Autodesk Inventor part; units mm, degrees
ref_plane "YZ Plane" through (0, 0, 0) normal (1, 0, 0) x (0, 1, 0)
ref_plane "XZ Plane" through (0, 0, 0) normal (0, 1, 0) x (-1, 0, 0)
ref_plane "XY Plane" through (0, 0, 0) normal (0, 0, 1) x (1, 0, 0)
sketch "Sketch1" plane through (0, 0, 0) normal (0, 1, 0) x (-1, 0, 0)
  line L0 (70, 50) -> (-70, 50)
  line L1 (-70, 50) -> (-70, -50)
  line L2 (-70, -50) -> (70, -50)
  line L3 (70, -50) -> (70, 50)
  line L4 (70, 50) -> (-70, -50) construction
  line L5 (-70, 50) -> (70, -50) construction
  point P0 (0, 0)
  dimension "d0" = 140
  dimension "d1" = 100
extrude "Extrusion1" add sketch "Sketch1" along normal blind 3.125
sketch "Sketch9" plane through (0, 3.125, 0) normal (0, 1, 0) x (1, 0, 0)
  circle A0 centre (-1.7146, 21.2758) radius 10
  point P0 (0, 0)
  dimension "d41" = 20
extrude "Extrusion9" cut sketch "Sketch9" against normal blind 10
sketch "Sketch10" plane through (0, 3.125, 0) normal (0, 1, 0) x (1, 0, 0)
  circle A0 centre (-31.6428, 0) radius 2
  point P0 (0, 0)
  dimension "d44" = 4
extrude "Extrusion10" cut sketch "Sketch10" against normal blind 5
sketch "Sketch11" plane through (0, 3.125, 0) normal (0, 1, 0) x (1, 0, 0)
  circle A0 centre (20.6742, 0) radius 2
  point P0 (0, 0)
  dimension "d47" = 4
extrude "Extrusion11" cut sketch "Sketch11" against normal blind 5
sketch "Sketch15" plane through (0, 3.125, 0) normal (0, 1, 0) x (1, 0, 0)
  line L0 (-16.402, 10) -> (-13.247, 10)
  line L1 (-13.247, 10) -> (-13.247, -10)
  line L2 (-13.247, -10) -> (-16.402, -10)
  line L3 (-16.402, -10) -> (-16.402, 10)
  line L4 (-16.402, 10) -> (-13.247, -10) construction
  line L5 (-13.247, 10) -> (-16.402, -10) construction
  line L6 (61.753, 10) -> (64.908, 10)
  line L7 (64.908, 10) -> (64.908, -10)
  line L8 (64.908, -10) -> (61.753, -10)
  line L9 (61.753, -10) -> (61.753, 10)
  line L10 (61.753, 10) -> (64.908, -10) construction
  line L11 (64.908, 10) -> (61.753, -10) construction
  point P0 (0, 0)
  point P1 (-14.8245, 0)
  point P2 (63.3305, 0)
  dimension "d68" = 3.155
  dimension "d69" = 20
  dimension "d70" = 3.155
  dimension "d71" = 20
  dimension "d72" = 75
extrude "Extrusion14" cut sketch "Sketch15" against normal blind 3.125
sketch "Sketch16" plane through (0, 3.125, 0) normal (0, 1, 0) x (1, 0, 0)
  line L0 (-70, -50) -> (70, -50)
  line L1 (-70, 50) -> (-40.7108, 50)
  line L2 (-40.7108, 50) -> (-40.7108, -50)
  line L3 (-40.7108, -50) -> (-70, -50)
  line L4 (-70, -50) -> (-70, 50)
  point P0 (0, 0)
extrude "Extrusion15" cut sketch "Sketch16" against normal blind 3.125
properties part number "Base"
The listing builds one solid part. Answer for the finished solid, in the listing's coordinates (mm). A direction names the side the tool comes from. Give positions to 0.01 mm unless a question says otherwise; leave off trailing zeros. Order: outer loops, then holes, each group sorted by start corner. A loop starts at its lowest first (then second) coordinate and runs counter-clockwise, first axis right, second up. Notation, with made-up numbers: (68, 83) - (97, 83) arc R34 ccw to (97, 119) - close; hole circle Ø6 at (74.25, 86). An arc over 180 degrees is marked (long way). Use one line per item in the form item = value. Start each with the question number.
(1) Consider line 1 (X direction, y = 0.75, z = 0); line 2 (X direction, y = 2.4, z = -7.5); line 3 (Z direction, x = 1, y = 0.35). Determine where each line is inside the solid, lowest interval first. Write a range as from..to.
(2) For faces 1 (the flat face through (70, 2, 1)), 2 (the flat face through (-15, 2, 10)), determine the directions among +Z, -Z, +X, -X, +Y, -Y from which every point of the face is accessible in a straight line to the end or side of a thin tool.
(3) A cutting plane is placed at B-B, the plane y = 2.6. Write down the section's boundary in (x, z), then the cut area to 3 significant figures.
(4) The mould has two halves that part along Z. Classify faces 3 (the flat face through (63, 2, -10)), 4 (the flat face through (-40.711, 2, -1)), 5 (the flat face through (61.753, 2, 0)), 6 (the flat face through (14, 2, 50)): released by +Z, released by -Z, zero draft, split by the parting line, or undercut.
(5) A cutting plane is placed at A-A, the plane z = 6. Write down the section's boundary in (x, y) (3 decimals), then the cut area to 3 significant figures.
Ans:
q1.line_1 = -40.71..-33.64, -29.64..-16.4, -13.25..18.67, 22.67..61.75, 64.91..70
q1.line_2 = -40.71..-16.4, -13.25..61.75, 64.91..70
q1.line_3 = -50..-30.9, -11.65..50
q2.face_1 = +Z, -Z, +X, +Y, -Y
q2.face_2 = +Y, -Y
q3.outline = (-40.71, -50) - (70, -50) - (70, 50) - (-40.71, 50) - close; hole circle Ø4 at (-31.64, 0); hole (-16.4, -10) - (-13.25, -10) - (-13.25, 10) - (-16.4, 10) - close; hole circle Ø20 at (-1.71, -21.28); hole circle Ø4 at (20.67, 0); hole (61.75, -10) - (64.91, -10) - (64.91, 10) - (61.75, 10) - close
q3.area = 10,600 mm^2
q4.face_3 = undercut
q4.face_4 = zero draft
q4.face_5 = undercut
q4.face_6 = released by +Z
q5.outline = (-40.711, 0) - (-16.402, 0) - (-16.402, 3.125) - (-40.711, 3.125) - close; (-13.247, 0) - (61.753, 0) - (61.753, 3.125) - (-13.247, 3.125) - close; (64.908, 0) - (70, 0) - (70, 3.125) - (64.908, 3.125) - close
q5.area = 326 mm^2
